CAD build for the part. Positions are in the model's coordinates, mm. A direction names the side the tool comes from. Round coordinates to 2 decimals unless told otherwise and drop trailing zeros. Loops run counter-clockwise (first coordinate to the right, second up) from the corner with the lowest first, then second, coordinate; pieces in that order, holes last. Notation, with made-up numbers: M -4.5,-32.5 L 7.5,-32.5 A10 cw 7.5,-16.5 Z; hole C 10,-29 d5. An arc over 180 degrees is marked long. Use a Markdown table: item, result. Add a question column.
(1) Flat gauge pins, fed straight in: P1, Ø14.5, axis at y = -158, z = 9.5, coming from the +X side; P2, Ø11.5, axis at x = 37, y = -120.5, coming from the +Z side; P3, Ø14.5, axis at y = -197, z = 7.5, coming from the -X side. Where does each tip first touch, or does it go through?
(2) Which spindle directions (+Z, -Z, +X, -X, +Y, -Y) get a long thin tool onto all of the face, cutting with end or side? Do faces 1 (the face through (-27.345, -173, 5)), 2 (the face through (35, -173, -4)), 3 (the face through (26.345, -173, 10)). Say none if no direction does.
(3) Wall check: L1, parallel to X at y = -270, z = 12.25; L2, parallel to Z at x = 4, y = -182; L3, parallel to X at y = -134, z = 1.75. Give the ranges that are in metal, low to high.
(4) Band-saw the part on C-C, the plane x = -35. Write the cut outline in (y, z).
(5) Band-saw the part on D-D, the plane x = -18. Write the cut outline in (y, z), and give its area (3 significant figures).
(6) Band-saw the part on B-B, the plane y = -43. Write the cut outline in (x, z).
(7) Band-saw the part on A-A, the plane z = 11. Write the cut outline in (x, y), and give its area (3 significant figures).
from build123d import *

# Parameters (mm, degrees)
F1_DEPTH = 350


with BuildPart() as f1:
    # F0 (on Front) → F1 (new body)
    with BuildSketch(Plane.XZ):
        with BuildLine():
            Line((-9.656821, 5.487433), (-9.656821, 4.812567))
            ThreePointArc((-9.656821, 4.812567), (-9.65, 5.15), (-9.656821, 5.487433))
        make_face()
        with BuildLine():
            Line((-42, -14), (42, -14))
            Line((42, -14), (42, -4))
            Line((42, -4), (27.345447, -4))
            Line((27.345447, -4), (27.345447, 14))
            Line((27.345447, 14), (26.345447, 14))
            Line((26.345447, 14), (26.345447, 5.425711))
            ThreePointArc((26.345447, 5.425711), (17.987329, -3.19999), (9.655428, 5.451038))
            Line((9.655428, 5.451038), (9.655428, 14))
            Line((9.655428, 14), (5, 14))
            Line((5, 14), (5, -4))
            Line((5, -4), (-5, -4))
            Line((-5, -4), (-5, 14))
            Line((-5, 14), (-9.656821, 14))
            Line((-9.656821, 14), (-9.656821, 5.487433))
            ThreePointArc((-9.656821, 5.487433), (-9.65, 5.15), (-9.656821, 4.812567))
            ThreePointArc((-9.656821, 4.812567), (-18.316515, -3.193999), (-26.344766, 5.445596))
            Line((-26.344766, 5.445596), (-26.344766, 14))
            Line((-26.344766, 14), (-27.344766, 14))
            Line((-27.344766, 14), (-27.344766, -4))
            Line((-27.344766, -4), (-42, -4))
            Line((-42, -4), (-42, -14))
        make_face()
    extrude(amount=F1_DEPTH)


solid = f1.part
Return value:
| question | item | result |
|---|---|---|
| 1 | P1 | x = 27.35 |
| 1 | P2 | z = -4 |
| 1 | P3 | x = -27.34 |
| 2 | face 1 | +Z, -X, +Y, -Y |
| 2 | face 2 | +Z, +X, +Y, -Y |
| 2 | face 3 | +Z, +Y, -Y |
| 3 | L1 | -27.34 to -26.34, -9.66 to -5, 5 to 9.66, 26.35 to 27.35 |
| 3 | L2 | -14 to -4 |
| 3 | L3 | -27.34 to -25.63, -10.37 to -5, 5 to 10.37, 25.63 to 27.35 |
| 4 | outline | M -350,-14 L 0,-14 L 0,-4 L -350,-4 Z |
| 5 | outline | M -350,-14 L 0,-14 L 0,-3.2 L -350,-3.2 Z |
| 5 | area | 3,780 mm^2 |
| 6 | outline | M -42,-14 L 42,-14 L 42,-4 L 27.35,-4 L 27.35,14 L 26.35,14 L 26.35,5.43 A8.35 cw long 9.66,5.45 L 9.66,14 L 5,14 L 5,-4 L -5,-4 L -5,14 L -9.66,14 L -9.66,4.81 A8.35 cw -26.34,5.45 L -26.34,14 L -27.34,14 L -27.34,-4 L -42,-4 Z |
| 7 | outline | M -27.34,-350 L -26.34,-350 L -26.34,0 L -27.34,0 Z; M -9.66,-350 L -5,-350 L -5,0 L -9.66,0 Z; M 5,-350 L 9.66,-350 L 9.66,0 L 5,0 Z; M 26.35,-350 L 27.35,-350 L 27.35,0 L 26.35,0 Z |
| 7 | area | 3,960 mm^2 |
